```python
from build123d import *

# Parameters (mm, degrees)
F0_W     = 210
F0_H     = 170
F1_DEPTH = 30
F2_T     = -3
F3_W     = 12
F3_H     = 3.5
F3_W_2   = 14
F3_H_2   = 2.4
F3_W_3   = 5
F3_H_3   = 2.2
F3_W_4   = 13.34
F3_H_4   = 6
F3_W_5   = 6
F3_H_5   = 4
F4_DEPTH = 25
F5_W     = 5.91059
F5_H     = 73.586922
F6_DEPTH = 25


with BuildPart() as f1:
    # F0 (on Top) → F1 (new body)
    with BuildSketch(Plane.XY):
        Rectangle(F0_W, F0_H)
    extrude(amount=F1_DEPTH)

    # F2
    f2_openings = [f1.faces().sort_by_distance(p)[0] for p in [
        (0, 0, 30),
    ]]
    offset(amount=F2_T, openings=f2_openings)

    # F3 (on face) → F4 (cut)
    with BuildSketch(Plane(origin=(0, 85, 0), x_dir=(-1, 0, 0), z_dir=(0, 1, 0))):
        with Locations((44, 5.812878)):
            Rectangle(F3_W, F3_H)
        with Locations((19.7, 5.812878)):
            Rectangle(F3_W_2, F3_H)
        with Locations((0, 6.362878)):
            Rectangle(F3_W_2, F3_H_2)
        with Locations((-70.5, 6.462878)):
            Rectangle(F3_W_3, F3_H_3)
        with Locations((43.881843, 20.562878)):
            Rectangle(F3_W_4, F3_H_4)
        with Locations((23.881843, 20.562878)):
            Rectangle(F3_W_4, F3_H_4)
        with Locations((67.530297, 20.562878)):
            Rectangle(F3_W_5, F3_H_5)
    extrude(amount=-F4_DEPTH, mode=Mode.SUBTRACT)

    # F5 (on face) → F6 (cut)
    with BuildSketch(Plane(origin=(0, 0, 0), x_dir=(1, 0, 0), z_dir=(0, 0, -1))):
        with Locations((-93.378186, 43.943266)):
            Rectangle(F5_W, F5_H)
        with Locations((-93.378186, -43.943266)):
            Rectangle(F5_W, F5_H)
        with Locations((-83.678186, 43.943266)):
            Rectangle(F5_W, F5_H)
        with Locations((-83.678186, -43.943266)):
            Rectangle(F5_W, F5_H)
        with Locations((-73.978186, 43.943266)):
            Rectangle(F5_W, F5_H)
        with Locations((-73.978186, -43.943266)):
            Rectangle(F5_W, F5_H)
        with Locations((-64.278186, 43.943266)):
            Rectangle(F5_W, F5_H)
        with Locations((-64.278186, -43.943266)):
            Rectangle(F5_W, F5_H)
        with Locations((-54.578186, 43.943266)):
            Rectangle(F5_W, F5_H)
        with Locations((-54.578186, -43.943266)):
            Rectangle(F5_W, F5_H)
        with Locations((-44.878186, 43.943266)):
            Rectangle(F5_W, F5_H)
        with Locations((-44.878186, -43.943266)):
            Rectangle(F5_W, F5_H)
        with Locations((-35.178186, 43.943266)):
            Rectangle(F5_W, F5_H)
        with Locations((-35.178186, -43.943266)):
            Rectangle(F5_W, F5_H)
        with Locations((-25.478186, 43.943266)):
            Rectangle(F5_W, F5_H)
        with Locations((-25.478186, -43.943266)):
            Rectangle(F5_W, F5_H)
        with Locations((-15.778186, 43.943266)):
            Rectangle(F5_W, F5_H)
        with Locations((-15.778186, -43.943266)):
            Rectangle(F5_W, F5_H)
        with Locations((93.378186, 43.943266)):
            Rectangle(F5_W, F5_H)
        with Locations((83.678186, 43.943266)):
            Rectangle(F5_W, F5_H)
        with Locations((73.978186, 43.943266)):
            Rectangle(F5_W, F5_H)
        with Locations((64.278186, 43.943266)):
            Rectangle(F5_W, F5_H)
        with Locations((54.578186, 43.943266)):
            Rectangle(F5_W, F5_H)
        with Locations((44.878186, 43.943266)):
            Rectangle(F5_W, F5_H)
        with Locations((35.178186, 43.943266)):
            Rectangle(F5_W, F5_H)
        with Locations((25.478186, 43.943266)):
            Rectangle(F5_W, F5_H)
        with Locations((15.778186, 43.943266)):
            Rectangle(F5_W, F5_H)
        with Locations((93.378186, -43.943266)):
            Rectangle(F5_W, F5_H)
        with Locations((83.678186, -43.943266)):
            Rectangle(F5_W, F5_H)
        with Locations((73.978186, -43.943266)):
            Rectangle(F5_W, F5_H)
        with Locations((64.278186, -43.943266)):
            Rectangle(F5_W, F5_H)
        with Locations((54.578186, -43.943266)):
            Rectangle(F5_W, F5_H)
        with Locations((44.878186, -43.943266)):
            Rectangle(F5_W, F5_H)
        with Locations((35.178186, -43.943266)):
            Rectangle(F5_W, F5_H)
        with Locations((25.478186, -43.943266)):
            Rectangle(F5_W, F5_H)
        with Locations((15.778186, -43.943266)):
            Rectangle(F5_W, F5_H)
    extrude(amount=-F6_DEPTH, mode=Mode.SUBTRACT)


solid = f1.part
```
Check sheet for the modelled part. Datum: model origin and axes. Units: mm. A direction names the side the tool comes from. Coordinates: 2 decimals unless noted, no trailing zeros. Order: outer loops, then holes, each group sorted by start corner. A loop starts at its lowest first (then second) coordinate and runs counter-clockwise, first axis right, second up. Notation, with made-up numbers: M 24,-35.75 L 83,-35.75 A22 ccw 83,-23.75 Z; hole C -24,55 d5. An arc over 180 degrees is marked long. Write each question's results on one line, items separated by ' | '. Start each with the question number.
1. Go/stop test with a flat-tipped pin: P1, Ø6, axis at x = -36.5, y = -12.5, coming from the +Z side. Record where the tip stops, or that it passes through.
2. Cross-section at C-C on z = 15.25. Record the cut outline in (x, y).
3. Access from +Z, -Z, +X, -X, +Y, -Y to the whole of each face (thin tool, end or side, straight path). Record for faces 1 (the face through (-1, 1, 0)), 2 (the face through (-1, 1, 3)).
4. Cross-section at B-B on x = -3.5. Record the cut outline in (y, z).
5. Material ranges on probe 1 along Y at (x, z) = (-51.5, 3.75); probe 2 along X at (y, z) = (-73, 16.5); probe 3 along Z at (x, y) = (90, 74.5), recorded low to high.
6. Mould release check, pull along X, two halves, no side actions. Record for faces 3 (the face through (-1, -82, 16)), 4 (the face through (-105, -1, 15)), 5 (the face through (-0.5, 82.2, 30)): +X half, -X half, draft (parallel to the pull), parting line (faces both ways), or undercut.
7. Cross-section at A-A on x = -83. Record the cut outline in (y, z), and give its area (3 significant figures).
8. Cross-section at D-D on y = -75. State how many separate pieces and enclosed holes the cut face has, and give its area (3 significant figures).
Checks:
1) P1: stops at z = 3
2) outline: M -105,-85 L 105,-85 L 105,85 L -105,85 Z; hole M -102,-82 L 102,-82 L 102,82 L -102,82 Z
3) face 1: -Z, +X, -X, +Y, -Y | face 2: +Z
4) outline: M -85,0 L 85,0 L 85,5.16 L 82,5.16 L 82,3 L -82,3 L -82,30 L -85,30 Z; M 82,7.56 L 85,7.56 L 85,30 L 82,30 Z
5) probe 1: y = -85 to -82, 82 to 85 | probe 2: x = -105 to -102, 102 to 105 | probe 3: z = 0 to 3
6) face 3: undercut | face 4: -X half | face 5: draft
7) outline: M -85,0 L -80.74,0 L -80.74,3 L -82,3 L -82,30 L -85,30 Z; M -7.15,0 L 7.15,0 L 7.15,3 L -7.15,3 Z; M 80.74,0 L 85,0 L 85,30 L 82,30 L 82,3 L 80.74,3 Z | area: 230 mm²
8) separate pieces: 19 | enclosed holes: 0 | area: 473 mm²
